from build123d import *

# Parameters (mm, degrees)
F0_R     = 3.3655
F1_DEPTH = 2.558009
F2_R     = 4.1021
F3_DEPTH = 3.2
F4_R     = 2.3241
F5_DEPTH = 3.4544
F6_R     = 1.5875
F7_DEPTH = 7.62


with BuildPart() as f1:
    # F0 (on Top) → F1 (new body)
    with BuildSketch(Plane.XY):
        Circle(F0_R)
    extrude(amount=F1_DEPTH)

    # F2 (on face) → F3 (join)
    with BuildSketch(Plane(origin=(0, 0, 0), x_dir=(1, 0, 0), z_dir=(0, 0, -1))):
        Circle(F2_R)
    extrude(amount=F3_DEPTH)

    # F4 (on face) → F5 (cut)
    with BuildSketch(Plane(origin=(0, 0, -3.2), x_dir=(1, 0, 0), z_dir=(0, 0, -1))):
        Circle(F4_R)
    extrude(amount=-F5_DEPTH, mode=Mode.SUBTRACT)

    # F6 (on face) → F7 (cut)
    with BuildSketch(Plane.XY.offset(2.558009)):
        Circle(F6_R)
    extrude(amount=-F7_DEPTH, mode=Mode.SUBTRACT)


solid = f1.part
Can you work these out from the model? Positions are in its coordinate system, mm. A direction names the side the tool comes from. Coordinates: 2 decimals unless noted, no trailing zeros. Write each loop counter-clockwise with the first axis right and the second up, starting at its lowest first coordinate (ties: lowest second). Pieces come first, ordered by that corner, then holes.
Q1. Imagine slicing it at C-C, the plane z = 2.2. List the corners of the cut face in (x, y) for me (1 decimal), plus the area to 3 significant figures.
Results found:
outline: circle Ø6.7 at (0, 0); hole circle Ø3.2 at (0, 0)
area: 27.7 mm2
Q2. Imagine slicing it at A-A, the plane y = 0. List the corners of the cut face in (x, z) for me.
Results found:
outline: (-4.1, -3.2) - (-2.32, -3.2) - (-2.32, 0.25) - (-1.59, 0.25) - (-1.59, 2.56) - (-3.37, 2.56) - (-3.37, 0) - (-4.1, 0) - close; (1.59, 0.25) - (2.32, 0.25) - (2.32, -3.2) - (4.1, -3.2) - (4.1, 0) - (3.37, 0) - (3.37, 2.56) - (1.59, 2.56) - close
Q3. Which directions (+Z, -Z, +X, -X, +Y, -Y) give clear straight access to the entire face, cutting with the end or side of a thin tool? Please do faces 5 (the face through (-2, -1, 2.558)), 6 (the face through (-3, -2, 0)).
Results found:
face 5: +Z, +X, -X, +Y, -Y
face 6: +Z
Q4. Please list where these lines run through material, in increasing order: L1, parallel to X at y = 0, z = -1.55; L2, parallel to Y at x = 0, z = 1.2.
Results found:
L1: x = -4.1 to -2.32, 2.32 to 4.1
L2: y = -3.37 to -1.59, 1.59 to 3.37
Q5. Imagine slicing it at D-D, the plane y = -2.5. List the corners of the cut face in (x, z) for me.
Results found:
outline: (-3.25, -3.2) - (3.25, -3.2) - (3.25, 0) - (2.25, 0) - (2.25, 2.56) - (-2.25, 2.56) - (-2.25, 0) - (-3.25, 0) - close
Q6. For P1, Ø3, axis at x = -0.5, y = 0, coming from the -Z side, with a flat end and sliding along its axis, tell me the tip position at first contact or that it passes through.
Results found:
P1: stops at z = 0.25
Q7. If we mould it in two halves opening along X, with no side actions, what happens to faces 1 (the face through (2, 2, -3.2)), 2 (the face through (0, 2, 0.254)), 3 (the face through (-0.5, 2.27, -1.5)), 4 (the face through (-2.67, -2.05, 1.26))? For each: +X half, -X half, draft (parallel to the pull), parting line (faces both ways), or undercut.
Results found:
face 1: draft
face 2: undercut
face 3: undercut
face 4: parting line
